Check sheet for the modelled part. Datum: model origin and axes. Units: mm. Round coordinates to 2 decimals unless told otherwise and drop trailing zeros. Write each loop counter-clockwise with the first axis right and the second up, starting at its lowest first coordinate (ties: lowest second). Pieces come first, ordered by that corner, then holes.
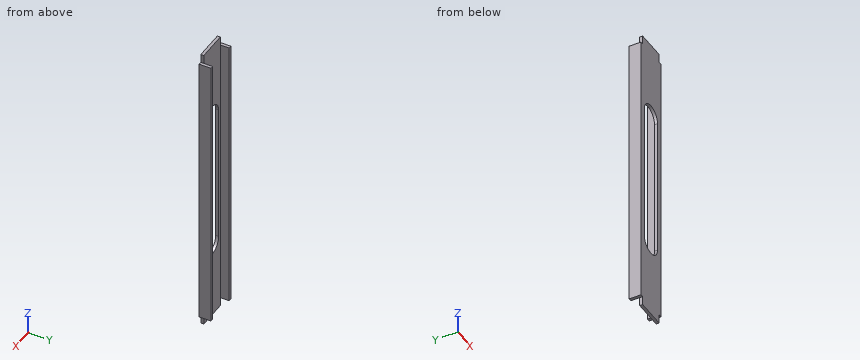
from build123d import *

# Parameters (mm, degrees)
BOSS_EXTRUDE1_DEPTH = 323.85
SKETCH2_W           = 9.525
SKETCH2_H           = 12.7
CUT_EXTRUDE1_DEPTH  = 3.175
CUT_EXTRUDE2_REACH  = 14.7


with BuildPart() as part:
    # Sketch1 → Boss-Extrude1 (new body)
    with BuildSketch(Plane.XY):
        Polygon((3.175, 3.175), (3.175, 12.7), (0, 12.7), (0, 0), (38.1, 0), (38.1, 12.7), (34.925, 12.7), (34.925, 3.175), align=None)
    extrude(amount=BOSS_EXTRUDE1_DEPTH)

    # Sketch2 → Cut-Extrude1 (cut)
    with BuildSketch(Plane.ZY):
        with Locations((319.0875, 6.35)):
            Rectangle(SKETCH2_W, SKETCH2_H)
        with Locations((4.7625, 6.35)):
            Rectangle(SKETCH2_W, SKETCH2_H)
    cut_extrude1 = extrude(amount=-CUT_EXTRUDE1_DEPTH, mode=Mode.SUBTRACT)

    # Mirror1: Cut-Extrude1 across plane
    add(cut_extrude1.mirror(Plane.ZY.offset(-19.05)), mode=Mode.SUBTRACT)

    # Sketch3 → Cut-Extrude2 (cut, up to next)
    with BuildSketch(Plane.XZ, mode=Mode.PRIVATE) as cut_extrude2_sk1:
        with BuildLine():
            Line((31.75, 238.125), (31.75, 85.725))
            ThreePointArc((31.75, 85.725), (19.05, 73.025), (6.35, 85.725))
            Line((6.35, 85.725), (6.35, 238.125))
            ThreePointArc((6.35, 238.125), (19.05, 250.825), (31.75, 238.125))
        make_face()
    cut_extrude2_tool1 = extrude(cut_extrude2_sk1.sketch, amount=-CUT_EXTRUDE2_REACH, mode=Mode.PRIVATE) & part.part
    add(cut_extrude2_tool1.solids().sort_by_distance((19.05, 0, 161.925))[0], mode=Mode.SUBTRACT)


solid = part.part
1. Scan lines: line 1 along X through (y, z) = (7, 191) (3 decimals); line 2 along X through (y, z) = (2.25, 111.5); line 3 along Z through (x, y) = (9.5, 1). Record each from-to range of solid material in increasing order.
2. Go/stop test with flat-tipped pins: pin 1 (2.5 mm diameter, centred on x = 1, y = 7, fed in from +Z) (3 decimals); pin 2 (6 mm diameter, centred on x = 11.5, z = 258, fed in from +Y) (3 decimals); pin 3 (1 mm diameter, centred on x = 36, y = 8, fed in from -Z) (3 decimals); pin 4 (1.6 mm diameter, centred on y = 2, z = 182.5, fed in from -X). Record where each tip stops, or that it passes through.
3. Sectioned sample at C-C, the plane z = 169. Enter the section's corners in (x, y) (3 decimals), plus the area to 3 significant figures.
4. Sectioned sample at A-A, the plane x = 19.05. Enter the section's corners in (y, z) (3 decimals).
5. Sectioned sample at B-B, the plane y = 9.25. Enter the section's corners in (x, z) (3 decimals).
Computed values:
1. line 1: x = 0 to 3.175, 34.925 to 38.1
1. line 2: x = 0 to 6.35, 31.75 to 38.1
1. line 3: z = 0 to 77.35, 246.5 to 323.85
2. pin 1: stops at z = 314.325
2. pin 2: stops at y = 3.175
2. pin 3: stops at z = 9.525
2. pin 4: stops at x = 0
3. outline: (0, 0) - (6.35, 0) - (6.35, 3.175) - (3.175, 3.175) - (3.175, 12.7) - (0, 12.7) - close; (31.75, 0) - (38.1, 0) - (38.1, 12.7) - (34.925, 12.7) - (34.925, 3.175) - (31.75, 3.175) - close
3. area: 101 mm2
4. outline: (0, 0) - (3.175, 0) - (3.175, 73.025) - (0, 73.025) - close; (0, 250.825) - (3.175, 250.825) - (3.175, 323.85) - (0, 323.85) - close
5. outline: (0, 9.525) - (3.175, 9.525) - (3.175, 314.325) - (0, 314.325) - close; (34.925, 9.525) - (38.1, 9.525) - (38.1, 314.325) - (34.925, 314.325) - close
